Autodesk Inventor part; units mm, degrees
ref_plane "YZ Plane" through (0, 0, 0) normal (1, 0, 0) x (0, 1, 0)
ref_plane "XZ Plane" through (0, 0, 0) normal (0, 1, 0) x (-1, 0, 0)
ref_plane "XY Plane" through (0, 0, 0) normal (0, 0, 1) x (1, 0, 0)
sketch "Sketch1" plane through (0, 0, 0) normal (0, 1, 0) x (-1, 0, 0)
  line L0 (51.25, 0) -> (-51.25, 0)
  line L1 (-51.25, 0) -> (-51.25, 4.75)
  line L2 (-51.25, 6) -> (51.25, 6) construction
  line L3 (51.25, 6) -> (51.25, 4.75) construction
  line L4 (50, 6) -> (-50, 6)
  line L5 (-50, 6) -> (-51.25, 4.75)
  line L6 (50, 6) -> (51.25, 4.75)
  line L7 (51.25, 4.75) -> (51.25, 0)
  line L8 (-51.25, 4.75) -> (-51.25, 6) construction
  line L9 (47.5, -5.889) -> (44.95, -4.4167)
  line L10 (44.95, -4.4167) -> (44.95, -1.4722)
  line L11 (44.95, -1.4722) -> (47.5, 0)
  line L12 (47.5, 0) -> (50.05, -1.4722)
  line L13 (50.05, -1.4722) -> (50.05, -4.4167)
  line L14 (50.05, -4.4167) -> (47.5, -5.889)
  line L15 (47.5, -2.9445) -> (-47.5, -2.9445) construction
  line L16 (51.25, 0) -> (51.25, -5.0477)
  line L17 (51.25, -5.0477) -> (50.65, -5.6477)
  line L18 (50.65, -5.6477) -> (49.65, -4.6477)
  line L19 (50.05, -2.9445) -> (51.25, -2.9445) construction
  line L20 (45.35, -4.6477) -> (44.35, -5.6477)
  line L21 (44.35, -5.6477) -> (43.75, -5.0477)
  line L22 (43.75, -5.0477) -> (43.75, 0)
  line L23 (47.5, -5.889) -> (47.5, 0) construction
  line L24 (43.75, 0) -> (51.25, 0) construction
  point P0 (0, 0)
  point P1 (0, 0)
  point P2 (0, 0)
  point P3 (0, 6)
  point P4 (0, 6)
  point P5 (0, -2.9445)
  point P6 (50.65, -2.9445)
  dimension "d22" = 100
  dimension "d23" = 6
  dimension "d24" = 95
  dimension "d25" = 5.1
  dimension "d26" = 6
  dimension "d27" = 1.2
  dimension "d28" = 0.4
extrude "Extrusion1" add sketch "Sketch1" along normal blind 29.5 contours L0 L1 L5 L4 L6 L7
extrude "Extrusion3" add sketch "Sketch1" along normal blind 29.5 contours L16 L17 L18 L14 L13 L12 L0 | L11 L10 L9 L20 L21 L22 L0
mirror "Mirror1" about plane through (0, 0, 0) normal (1, 0, 0) of "Extrusion3"
sketch "Sketch2" plane through (41.9, 0, 0) normal (0, 0, -1) x (-1, 0, 0)
  line L0 (41.9, 29.5) -> (41.9, 0) construction
  line L1 (12.9, 20.5) -> (70.9, 20.5) construction
  line L2 (9.35, 22.5496) -> (12.9, 24.5992)
  line L3 (12.9, 24.5992) -> (16.45, 22.5496)
  line L4 (16.45, 22.5496) -> (16.45, 18.4504)
  line L5 (16.45, 18.4504) -> (12.9, 16.4008)
  line L6 (12.9, 16.4008) -> (9.35, 18.4504)
  line L7 (9.35, 18.4504) -> (9.35, 22.5496)
  line L8 (74.45, 22.5496) -> (74.45, 18.4504)
  line L9 (74.45, 18.4504) -> (70.9, 16.4008)
  line L10 (70.9, 16.4008) -> (67.35, 18.4504)
  line L11 (67.35, 18.4504) -> (67.35, 22.5496)
  line L12 (67.35, 22.5496) -> (70.9, 24.5992)
  line L13 (70.9, 24.5992) -> (74.45, 22.5496)
  line L14 (-1.85, 0) -> (85.65, 0) construction
  line L15 (-1.85, 29.5) -> (85.65, 29.5) construction
  point P0 (41.9, 20.5)
  point P1 (41.9, 14.75)
  dimension "d9" = 58
  dimension "d10" = 7.1
  dimension "d34" = 9
extrude "Extrusion2" cut sketch "Sketch2" against normal blind 5
hole "Hole1" at (29, 20.5, 0) at (-29, 20.5, 0) direction (0, 0, 1) diameter 3.9 end through all
chamfer "Chamfer1" distance 1 angle 45 2 edges at (-43.75, 14.75, 0) (43.75, 14.75, 0)
properties part number "switch_mount"
Check sheet for the modelled part. Datum: model origin and axes. Units: mm. A direction names the side the tool comes from. Round coordinates to 2 decimals unless told otherwise and drop trailing zeros. Loops run counter-clockwise (first coordinate to the right, second up) from the corner with the lowest first, then second, coordinate; pieces in that order, holes last. Notation, with made-up numbers: M -26.5,83 L 11.5,83 A20 ccw 11.5,109 Z; hole C 68.25,23.5 d6. An arc over 180 degrees is marked long. Answer as a JSON object with one key per item and string values.
1. Gauge pin test, flat ends, axial feed: P1, Ø2, axis at x = -17, y = 20, coming from the -Z side; P2, Ø2, axis at x = 28.5, y = 20, coming from the -Z side; P3, Ø4.5, axis at x = -29, y = 20.5, coming from the -Z side. Record the tip position at first contact, or that the pin passes through.
Reply:
{"P1": "stops at z = 0", "P2": "passes through", "P3": "stops at z = 5"}
2. Scan lines: line 1 (X direction, y = 21, z = 3); line 2 (X direction, y = 24.75, z = -1.75); line 3 (Y direction, x = -29, z = 5.5). Record each from-to range of solid material in increasing order.
Reply:
{"line 1": "x = -51.25 to -32.55, -25.45 to 25.45, 32.55 to 51.25", "line 2": "x = -51.25 to -50.05, -44.95 to -43.75, 43.75 to 44.95, 50.05 to 51.25", "line 3": "y = 0 to 18.55, 22.45 to 29.5"}
3. Section check A-A (z = 1.25). Record the boundary of the cut face in (x, y), plus the area to 3 significant figures.
Reply:
{"outline": "M -51.25,0 L 51.25,0 L 51.25,29.5 L -51.25,29.5 Z; hole M -32.55,18.45 L -29,16.4 L -25.45,18.45 L -25.45,22.55 L -29,24.6 L -32.55,22.55 Z; hole M 25.45,18.45 L 29,16.4 L 32.55,18.45 L 32.55,22.55 L 29,24.6 L 25.45,22.55 Z", "area": "2,940 mm²"}
4. Mould release check, pull along Z, two halves, no side actions. Record for faces 4 (the flat face through (-1, 15, 6)), 5 (the flat face through (-50.05, 15, -3)), 6 (the flat face through (44.95, 15, -3)), 7 (the flat face through (-25.45, 20, 2)): pulls with the +Z half, pulls with the -Z half, needs draft (parallel to the pull), parting line crosses it, or undercut.
Reply:
{"face 4": "pulls with the +Z half", "face 5": "undercut", "face 6": "undercut", "face 7": "needs draft"}
5. Section check B-B (x = 41). Record the boundary of the cut face in (y, z), plus the area to 3 significant figures.
Reply:
{"outline": "M 0,0 L 29.5,0 L 29.5,6 L 0,6 Z", "area": "177 mm²"}
6. Access from +Z, -Z, +X, -X, +Y, -Y to the whole of each face (thin tool, end or side, straight path). Record for faces 1 (the flat face through (-51.25, 15, 0)), 2 (the flat face through (50.05, 15, -3)), 3 (the flat face through (30.8, 23.56, 2.46)).
Reply:
{"face 1": "+Z, -Z, -X, +Y, -Y", "face 2": "+Y, -Y", "face 3": "-Z"}
7. Section check C-C (y = 21). State how many separate pieces and enclosed holes the cut face has, plus the area to 3 significant figures.
Reply:
{"separate pieces": "3", "enclosed holes": "0", "area": "570 mm²"}
